Geometry check sheet. Reference: drawing and pictorial views, mm from the part's lowest x, y, z. Give positions to 0.01 mm unless a question says otherwise; leave off trailing zeros. Write each loop counter-clockwise with the first axis right and the second up, starting at its lowest first coordinate (ties: lowest second). Pieces come first, ordered by that corner, then holes. Notation, with made-up numbers: (-1, 0.5) -> (27, 0.5) arc R17 cw to (27, 6.5) -> close; hole circle Ø4 at (25, 65.25). An arc over 180 degrees is marked (long way). Use a Markdown table: item, result. Add a question column.
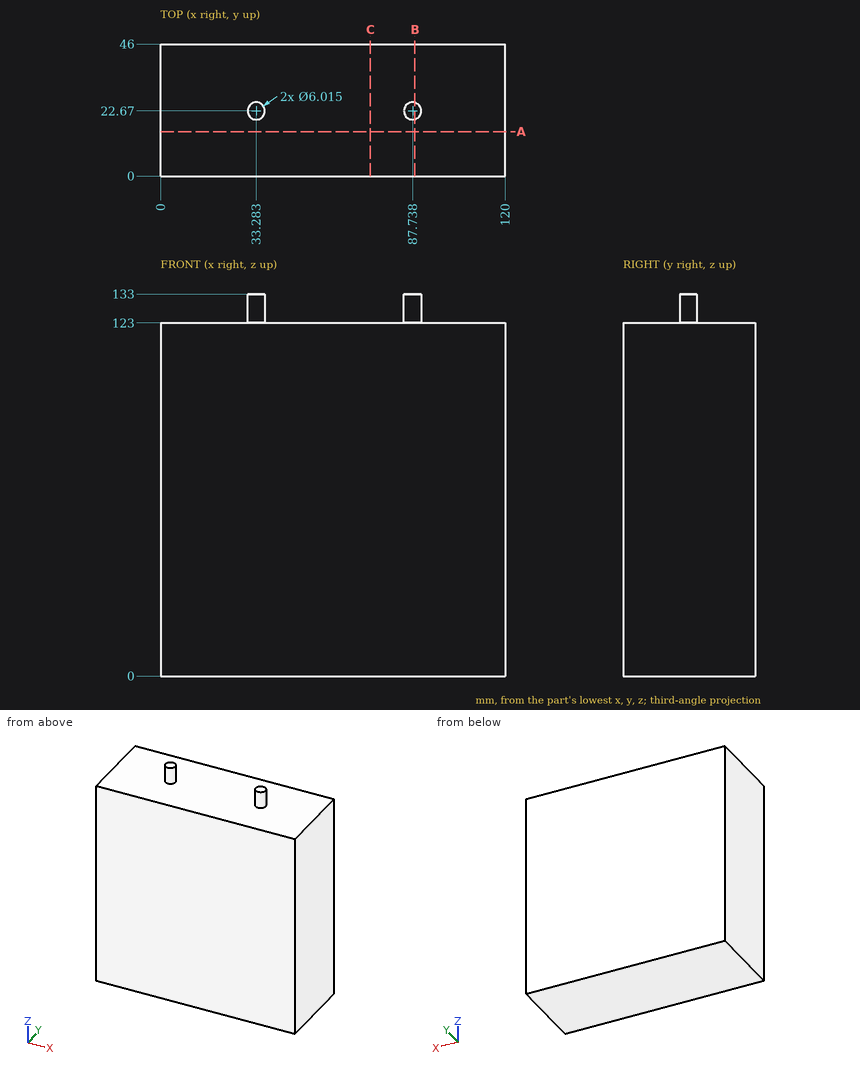
1) Material ranges on probe 1 along Z at (x, y) = (20.5, 22), recorded low to high. Write a range as [from, to].
2) Gauge pin test, flat end, axial feed: P1, Ø4, axis at x = 90.5, y = 6.5, coming from the +Z side. Record the tip position at first contact, or that the pin passes through.
3) Sectioned sample at C-C, the plane x = 73. Enter the section's corners in (y, z).
4) Sectioned sample at A-A, the plane y = 15.5. Enter the section's corners in (x, z).
5) Sectioned sample at B-B, the plane x = 88.5. Enter the section's corners in (y, z), and give its area (3 significant figures).
Check values:
| question | item | result |
|---|---|---|
| 1 | probe 1 | [0, 123] |
| 2 | P1 | z = 123 |
| 3 | outline | (0, 0) -> (46, 0) -> (46, 123) -> (0, 123) -> close |
| 4 | outline | (0, 0) -> (120, 0) -> (120, 123) -> (0, 123) -> close |
| 5 | outline | (0, 0) -> (46, 0) -> (46, 123) -> (25.58, 123) -> (25.58, 133) -> (19.76, 133) -> (19.76, 123) -> (0, 123) -> close |
| 5 | area | 5,720 mm² |
